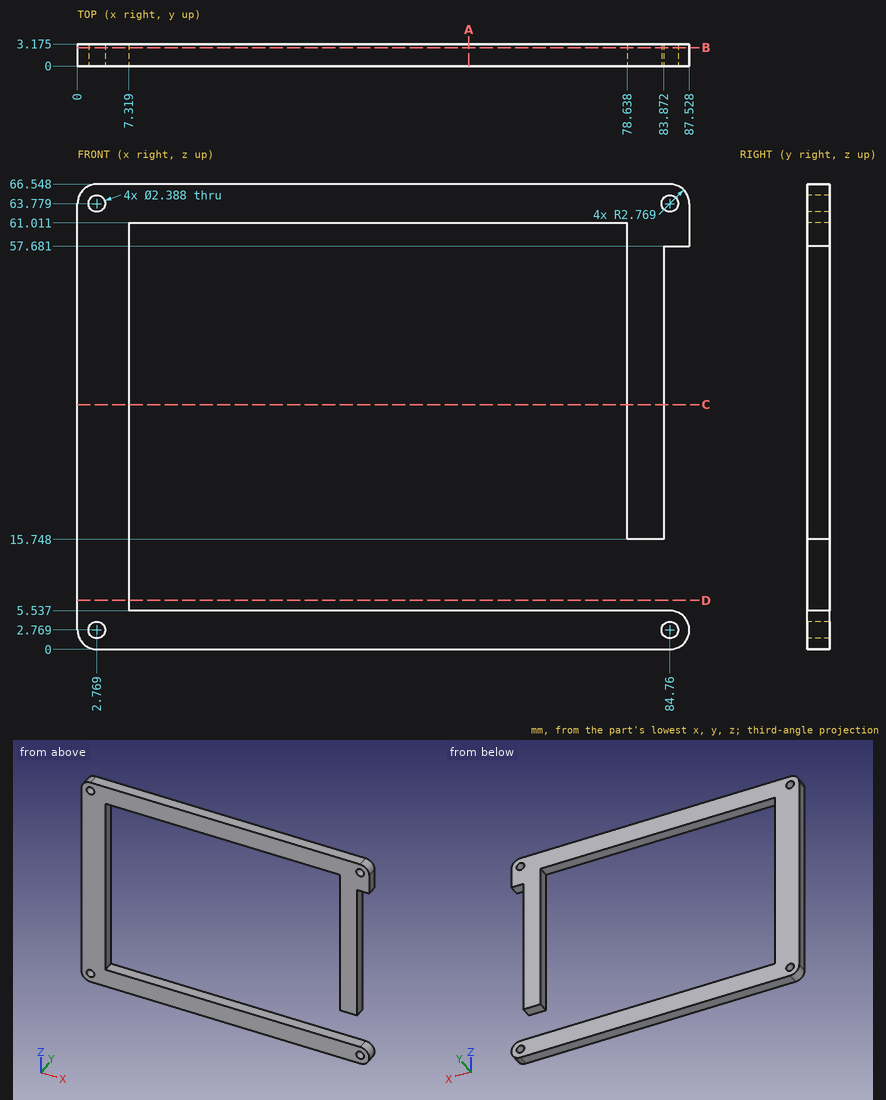
Verification items for this drawing (mm, ordinates from the low corner). Give positions to 0.01 mm unless a question says otherwise; leave off trailing zeros. Write each loop counter-clockwise with the first axis right and the second up, starting at its lowest first coordinate (ties: lowest second). Pieces come first, ordered by that corner, then holes. Notation, with made-up numbers: (74, 13.5) - (97, 13.5) arc R25 ccw to (97, 47.5) - close; hole circle Ø8 at (37, 84). An arc over 180 degrees is marked (long way). Answer as CSV lines item,"result". Start each with the question number.
1. Sectioned sample at A-A (x = 56). Record the boundary of the cut face in (y, z) (1 decimal).
2. Sectioned sample at C-C (z = 35). Record the boundary of the cut face in (x, y) (1 decimal).
3. Depth check by flat-ended pin: pin 1 (1.5 mm diameter, centred on y = 2.5, z = 40, fed in from -X); pin 2 (1.6 mm diameter, centred on y = 2, z = 28, fed in from +X); pin 3 (1.6 mm diameter, centred on x = 86.5, y = 1.5, fed in from -Z) (1 decimal). Enter the tip coordinate at first touch or a pass-through.
4. Sectioned sample at B-B (y = 2.65). Record the boundary of the cut face in (x, z), then the cut area to 3 significant figures.
5. Sectioned sample at D-D (z = 7). Record the boundary of the cut face in (x, y) (1 decimal).
6. Thickness scan on line 1 (Z direction, x = 19, y = 2.1); line 2 (Z direction, x = 82.5, y = 0.4); line 3 (X direction, y = 1.95, z = 47). Record the ranges inside material, lowest first.
Derived:
1,outline,"(0, 0) - (3.2, 0) - (3.2, 5.5) - (0, 5.5) - close; (0, 61) - (3.2, 61) - (3.2, 66.5) - (0, 66.5) - close"
2,outline,"(0, 0) - (7.3, 0) - (7.3, 3.2) - (0, 3.2) - close; (78.6, 0) - (83.9, 0) - (83.9, 3.2) - (78.6, 3.2) - close"
3,pin 1,"x = 0"
3,pin 2,"x = 83.87"
3,pin 3,"z = 0.2"
4,outline,"(0, 2.77) arc R2.77 ccw to (2.77, 0) - (84.76, 0) arc R2.77 ccw to (84.76, 5.54) - (7.32, 5.54) - (7.32, 61.01) - (78.64, 61.01) - (78.64, 15.75) - (83.87, 15.75) - (83.87, 57.68) - (87.53, 57.68) - (87.53, 63.78) arc R2.77 ccw to (84.76, 66.55) - (2.77, 66.55) arc R2.77 ccw to (0, 63.78) - close; hole circle Ø2.39 at (2.77, 2.77); hole circle Ø2.39 at (2.77, 63.78); hole circle Ø2.39 at (84.76, 2.77); hole circle Ø2.39 at (84.76, 63.78)"
4,area,"1,600 mm²"
5,outline,"(0, 0) - (7.3, 0) - (7.3, 3.2) - (0, 3.2) - close"
6,line 1,"0 to 5.54, 61.01 to 66.55"
6,line 2,"0 to 5.54, 15.75 to 66.55"
6,line 3,"0 to 7.32, 78.64 to 83.87"
